The model under review builds one solid part; all positions refer to its coordinate system, in mm. A direction names the side the tool comes from. Round coordinates to 2 decimals unless told otherwise and drop trailing zeros. Order: outer loops, then holes, each group sorted by start corner. A loop starts at its lowest first (then second) coordinate and runs counter-clockwise, first axis right, second up. Notation, with made-up numbers: (-14.5, -15.5) -> (4.5, -15.5) arc R35 cw to (4.5, 17.5) -> close; hole circle Ø2 at (10.5, 2). An arc over 180 degrees is marked (long way). Return JSON: item names as keys, results as strings. Group by question number.
from build123d import *

# Parameters (mm, degrees)
SKETCH_1_R          = 55
EXTRUDE_1_DEPTH     = 10
SKETCH_2_R          = 25
EXTRUDE_2_DEPTH     = 35
SKETCH_3_R          = 25
SKETCH_3_R_2        = 15
EXTRUDE_3_DEPTH     = 25
SKETCH_6_R          = 35.302710026
CUT_EXTRUDE_2_DEPTH = 10


with BuildPart() as part:
    # 草图1 → 凸台-拉伸1 (new body)
    with BuildSketch(Plane.XY):
        Circle(SKETCH_1_R)
    extrude(amount=EXTRUDE_1_DEPTH)

    # 草图2 → 凸台-拉伸2 (add)
    with BuildSketch(Plane(origin=(0, 0, 0), x_dir=(-1, 0, 0), z_dir=(0, 0, -1))):
        with Locations(Location((0, 0, 0), (0, 0, 180))):
            Circle(SKETCH_2_R)
    extrude(amount=EXTRUDE_2_DEPTH)

    # 草图3 → 凸台-拉伸3 (add, symmetric)
    # profile 1 of 2: a face of its own
    with BuildSketch(Plane(origin=(0, 0, 0), x_dir=(0, 0, -1), z_dir=(1, 0, 0))):
        with BuildLine():
            Line((-67.276717973, -81.520178774), (-10, -47.656713047))
            Line((-10, -47.656713047), (-10, 26.1722221))
            Line((-10, 26.1722221), (-95.356612975, -40.272495395))
            ThreePointArc((-95.356612975, -40.272495395), (-69.020822535, -37.539865045), (-55, -60))
            ThreePointArc((-55, -60), (-58.285004597, -72.387855935), (-67.276717973, -81.520178774))
        make_face()
    # profile 2 of 2: a face of its own
    with BuildSketch(Plane(origin=(0, 0, 0), x_dir=(0, 0, -1), z_dir=(1, 0, 0))):
        with Locations((-80, -60)):
            Circle(SKETCH_3_R)
        with Locations((-80, -60)):
            Circle(SKETCH_3_R_2, mode=Mode.SUBTRACT)
    extrude(amount=EXTRUDE_3_DEPTH, both=True)

    # 草图6 → 切除-拉伸2 (cut, symmetric)
    with BuildSketch(Plane(origin=(0, 0, 0), x_dir=(0, 0, -1), z_dir=(1, 0, 0))):
        with Locations((-80, -60)):
            Circle(SKETCH_6_R)
    extrude(amount=CUT_EXTRUDE_2_DEPTH, both=True, mode=Mode.SUBTRACT)


solid = part.part
Item 1: Wall thickness on line 1 along X through (y, z) = (-42, 71.5); line 2 along X through (y, z) = (-11.5, 34.5); line 3 along Z through (x, y) = (28.5, -2): over which ranges is each line inside the solid? List them lowest first.
Item 2: The part is to be moulded in two halves that separate along Z. For faces 5 (the face through (-17.6, -73.31, 73.08)), 6 (the face through (17.6, -73.63, 100.96)), 7 (the face through (10, -48, 69)), say which applies: +Z half, -Z half, draft (parallel to the pull), parting line (faces both ways), or undercut.
Item 3: Consider section A-A on y = -60. State the section outline as (x, z) points, plus the area to 3 significant figures.
Item 4: For faces 1 (the face through (-25, -29, 48)), 2 (the face through (0.14, -40.483, 50.583)), 3 (the face through (25, -29, 48)), 4 (the face through (11, -24, 0)), list the 3-axis set-ups (+Z, -Z, +X, -X, +Y, -Y) from which the entire face can be reached by the end or side of a thin tool; tool diameter is ignored.
Item 5: Consider section D-D on x = 2.5. State the section outline as (y, z) points.
Item 6: Consider section B-B on z = 80. State the section outline as (x, y) points, plus the area to 3 significant figures.
Item 7: Insertion check: pin 1 Ø2 at (x, z) = (-3.5, 29.5) entering from -Y; pin 2 Ø12 at (x, z) = (3, -19.5) entering from -Y; pin 3 Ø18 at (y, z) = (-60, 80) entering from +X; pin 4 Ø6 at (x, z) = (-43.5, 11) entering from +Y. Each pin has a flat end and moves straight along its axis. Give the tip position at first contact, or say it passes through.
Item 8: Consider section C-C on x = -23. State the section outline as (y, z) points.
Values:
{
 "1": {"line 1": "-25 to -10, 10 to 25", "line 2": "-25 to 25", "line 3": "0 to 10"},
 "2": {"face 5": "undercut", "face 6": "parting line", "face 7": "draft"},
 "3": {"outline": "(-25, 30.88) -> (25, 30.88) -> (25, 65) -> (10, 65) -> (10, 44.7) -> (-10, 44.7) -> (-10, 65) -> (-25, 65) -> close; (-25, 95) -> (-10, 95) -> (-10, 105) -> (-25, 105) -> close; (10, 95) -> (25, 95) -> (25, 105) -> (10, 105) -> close", "area": "1,600 mm^2"},
 "4": {"face 1": "+Z, -X, +Y, -Y", "face 2": "+Z", "face 3": "+Z, +X, +Y, -Y", "face 4": "-Z"},
 "5": {"outline": "(-68.83, 45.82) -> (-47.66, 10) -> (-54.94, 10) -> (-54.94, 0) -> (-24.87, 0) -> (-24.87, -35) -> (24.87, -35) -> (24.87, 0) -> (54.94, 0) -> (54.94, 10) -> (26.17, 10) -> (-24.96, 75.69) arc R35.3 cw to start"},
 "6": {"outline": "(-25, -85) -> (-10, -85) -> (-10, -75) -> (-25, -75) -> close; (-25, -45) -> (-10, -45) -> (-10, -28.32) -> (-25, -28.32) -> close; (10, -85) -> (25, -85) -> (25, -75) -> (10, -75) -> close; (10, -45) -> (25, -45) -> (25, -28.32) -> (10, -28.32) -> close", "area": "800 mm^2"},
 "7": {"pin 1": "y = -59.78", "pin 2": "y = -25", "pin 3": "through", "pin 4": "y = 37.02"},
 "8": {"outline": "(-81.52, 67.28) -> (-47.66, 10) -> (-49.96, 10) -> (-49.96, 0) -> (-9.8, 0) -> (-9.8, -35) -> (9.8, -35) -> (9.8, 0) -> (49.96, 0) -> (49.96, 10) -> (26.17, 10) -> (-40.27, 95.36) arc R25 ccw to start; hole circle Ø30 at (-60, 80)"}
}
